from build123d import *

# Parameters (mm, degrees)
F1_DEPTH  = 16
F2_W      = 70
F2_H      = 3
F3_DEPTH  = 2
F4_W      = 50
F4_H      = 14
F5_DEPTH  = 2
F6_R      = 1
F9_DEPTH  = 2
F11_DEPTH = 38.001
F13_D     = 4
F14_R     = 3
F14_R_2   = 2
F15_DEPTH = 5
F16_R     = 3


# Not quite as in the source:
# - a pattern or mirror of a feature is missing from the dataset's text; its kind, count and spacing are read off the source's solid


with BuildPart() as f1:
    # F0 (on Front) → F1 (new body)
    with BuildSketch(Plane.XZ):
        with BuildLine():
            Line((94, 11), (0, 11))
            ThreePointArc((0, 11), (-11, 0), (0, -11))
            Line((0, -11), (19, -11))
            ThreePointArc((19, -11), (21.7981112342, -11.8562609251), (23.6378571429, -14.1317705916))
            ThreePointArc((23.6378571429, -14.1317705916), (44.801622976, -42.9310620406), (77.2062019292, -58.0057903986))
            ThreePointArc((77.2062019292, -58.0057903986), (83.2137047902, -59.1076967266), (88.1803617021, -62.6624973259))
            Line((88.1803617021, -62.6624973259), (89.3682949555, -61))
            ThreePointArc((89.3682949555, -61), (83.8961627896, -57.2250659611), (77.3621310458, -56))
            ThreePointArc((77.3621310458, -56), (45.985801942, -41.3156371935), (25.493, -13.3844788282))
            ThreePointArc((25.493, -13.3844788282), (22.9173557279, -10.1987652951), (19, -9))
            Line((19, -9), (0, -9))
            ThreePointArc((0, -9), (-9, 0), (0, 9))
            Line((0, 9), (94, 9))
            Line((94, 9), (94, 11))
        make_face()
    extrude(amount=F1_DEPTH)

    # F2 (on face) → F3 (join)
    with BuildSketch(Plane.XY.offset(11)):
        with Locations((59, -17.5)):
            Rectangle(F2_W, F2_H)
    extrude(amount=-F3_DEPTH)

    # F4 (on face) → F5 (join)
    with BuildSketch(Plane.XZ.offset(19)):
        with Locations((69, 4)):
            Rectangle(F4_W, F4_H)
    extrude(amount=-F5_DEPTH)

    # F6
    f6_edges = [f1.edges().sort_by_distance(p)[0] for p in [
        (59, -19, 11),
        (69, -17, 9),
    ]]
    fillet(f6_edges, radius=F6_R)

    # F7: F1 across plane


with BuildPart() as f1_1:
    add(f1.part)
    add(f1.part.mirror(Plane.XZ))

    # F8 (on face) → F9 (cut)
    with BuildSketch(Plane.XY.offset(11)):
        with BuildLine():
            Line((94, 12), (34, 12))
            ThreePointArc((34, 12), (22, 0), (34, -12))
            Line((34, -12), (94, -12))
            Line((94, -12), (94, 12))
        make_face()
    extrude(amount=-F9_DEPTH, mode=Mode.SUBTRACT)

    # F10 (on face) → F11 (cut, through all)
    with BuildSketch(Plane.XZ.offset(19)):
        with BuildLine():
            ThreePointArc((50, 5), (47, 2), (50, -1))
            Line((50, -1), (70, -1))
            ThreePointArc((70, -1), (73, 2), (70, 5))
            Line((70, 5), (50, 5))
        make_face()
    extrude(amount=-F11_DEPTH, mode=Mode.SUBTRACT)

    # F13 (through all)
    with Locations(Plane.XZ.offset(19)):
        with Locations((80, 3)):
            Hole(F13_D / 2)

    # F14 (on face) → F15 (join)
    with BuildSketch(Plane(origin=(0, -17, 0), x_dir=(-1, 0, 0), z_dir=(0, 1, 0))):
        with Locations((-80, 3)):
            Circle(F14_R)
        with Locations((-80, 3)):
            Circle(F14_R_2, mode=Mode.SUBTRACT)
    f15 = extrude(amount=F15_DEPTH)

    # F15_copies: F15 across plane
    add(f15.mirror(Plane.ZX))

    # F16
    f16_edges = [f1_1.edges().sort_by_distance(p)[0] for p in [
        (44, -18, -3),
        (44, 18, -3),
        (94, -18, -3),
        (94, 18, -3),
    ]]
    fillet(f16_edges, radius=F16_R)


solid = f1_1.part
Can you work these out from the model? Positions are in its coordinate system, mm. A direction names the side the tool comes from. Give positions to 0.01 mm unless a question says otherwise; leave off trailing zeros. Order: outer loops, then holes, each group sorted by start corner. A loop starts at its lowest first (then second) coordinate and runs counter-clockwise, first axis right, second up. Notation, with made-up numbers: M -25,-2.5 L 29,-2.5 A20 ccw 29,11.5 Z; hole C -33.75,5 d3. An arc over 180 degrees is marked long. Use a Markdown table: item, result. Add a question column.
Item 1: Will these pins go through, and if not, where does the flat tip stop? pin 1 (0.9 mm diameter, centred on y = 17.5, z = 6.5, fed in from -X); pin 2 (8 mm diameter, centred on x = 66.5, y = 7, fed in from +Z); pin 3 (12 mm diameter, centred on y = 7, z = -54.5, fed in from +X).
Item 2: We'd pull the mould along X, two halves only. Please class faces 4 (the cylindrical face through (78.092, 15.549, 3.601)), 5 (the cylindrical face through (93.1, 17.99, -2.14)), 6 (the flat face through (74, -19, 5)), 7 (the cylindrical face through (44.86, 17.99, -2.1)): +X half, -X half, draft (parallel to the pull), parting line (faces both ways), or undercut.
Item 3: For faces 1 (the cylindrical face through (73, -18, 2)), 2 (the flat face through (79, 12, 1)), 3 (the cylindrical face through (46.37, -0.22, -41.63)), which set-ups out of +Z, -Z, +X, -X, +Y, -Y let a thin tool reach every point of the face, with its end or its side?
Item 4: If I drill on L1, parallel to Z at x = 8, y = 2; L2, parallel to Y at x = 82, z = -2; L3, parallel to Z at x = 80, y = -13.3, over which ranges is the centre line in solid material (lowest first)? Write a range as [from, to].
Item 5: Suppose I cut it at B-B (y = 8.5). List the corners of the cut face in (x, z) for me (1 decimal), then the cut area to 3 significant figures.
Item 6: Suppose I cut it at A-A (x = 65). List the corners of the cut face in (y, z) for me.
Item 7: Suppose I cut it at C-C (x = 84.5). List the corners of the cut face in (y, z) for me.
Item 8: Suppose I cut it at D-D (z = 3). Count the separate pieces of the cut face and the enclosed holes in it, then the cut area to 4 significant figures.
Answer sheet:
| question | item | result |
|---|---|---|
| 1 | pin 1 | stops at x = 44 |
| 1 | pin 2 | stops at z = -51.42 |
| 1 | pin 3 | stops at x = 88.87 |
| 2 | face 4 | undercut |
| 2 | face 5 | +X half |
| 2 | face 6 | draft |
| 2 | face 7 | -X half |
| 3 | face 1 | +Y, -Y |
| 3 | face 2 | +Z, +X |
| 3 | face 3 | +X, +Y, -Y |
| 4 | L1 | z = [-11, -9], [9, 11] |
| 4 | L2 | y = [-19, -17], [17, 19] |
| 4 | L3 | z = [-58.18, -56.16], [0, 1], [5, 6], [9, 11] |
| 5 | outline | M 0,-11 L 19,-11 A5 cw 23.6,-14.1 A72 ccw 77.2,-58 A14 cw 88.2,-62.7 L 89.4,-61 A16 ccw 77.4,-56 A70 cw 25.5,-13.4 A7 ccw 19,-9 L 0,-9 A9 cw 0,9 L 25.5,9 L 25.5,11 L 0,11 A11 ccw Z |
| 5 | area | 334 mm² |
| 6 | outline | M -19,-3 L -17,-3 L -17,-1 L -19,-1 Z; M -19,5 L -17,5 L -17,8 A1 cw -16,9 L -12,9 L -12,11 L -18,11 A1 ccw -19,10 Z; M -16,-54.59 L 16,-54.59 L 16,-52.45 L -16,-52.45 Z; M 12,9 L 16,9 A1 cw 17,8 L 17,5 L 19,5 L 19,10 A1 ccw 18,11 L 12,11 Z; M 17,-3 L 19,-3 L 19,-1 L 17,-1 Z |
| 7 | outline | M -19,-3 L -17,-3 L -17,8 A1 cw -16,9 L -12,9 L -12,11 L -18,11 A1 ccw -19,10 Z; M -16,-59.73 L 16,-59.73 L 16,-57.49 L -16,-57.49 Z; M 12,9 L 16,9 A1 cw 17,8 L 17,-3 L 19,-3 L 19,10 A1 ccw 18,11 L 12,11 Z |
| 8 | separate pieces | 7 |
| 8 | enclosed holes | 0 |
| 8 | area | 168.5 mm² |
